Check sheet for the modelled part. Datum: model origin and axes. Units: mm. Round coordinates to 2 decimals unless told otherwise and drop trailing zeros. Loops run counter-clockwise (first coordinate to the right, second up) from the corner with the lowest first, then second, coordinate; pieces in that order, holes last. Notation, with made-up numbers: (71.5, -36) - (115.5, -36) arc R22 cw to (115.5, -2) - close; hole circle Ø6 at (-15.75, 38). An arc over 180 degrees is marked (long way). Answer in a Markdown table with one row per item. Add a question column.
(1) Thickness scan on line 1 along Y through (x, z) = (457, -11); line 2 along Y through (x, z) = (-60.5, -6.5); line 3 along X through (y, z) = (8.5, 6). Record the ranges inside material, lowest first.
(2) Gauge pin test, flat ends, axial feed: pin 1 (14.5 mm diameter, centred on x = -77, z = -15.5, fed in from +Y); pin 2 (3 mm diameter, centred on x = 212, y = 13, fed in from -Z); pin 3 (4 mm diameter, centred on y = 33, z = 10, fed in from -X). Record the tip position at first contact, or that the pin passes through.
(3) Cross-section at A-A on x = -276.5. Enter the section's corners in (y, z).
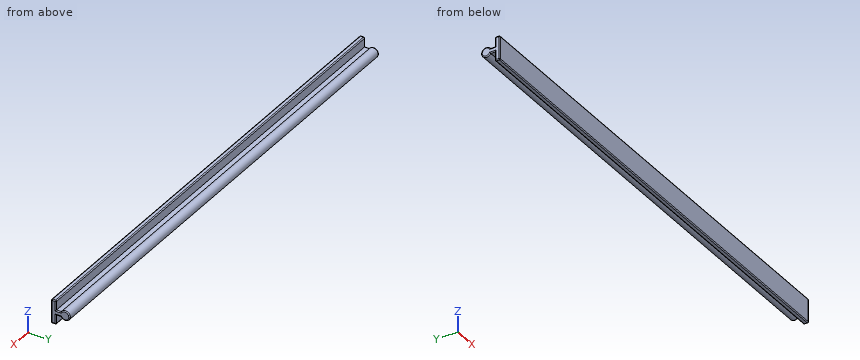
from build123d import *

# Parameters (mm, degrees)
BOSS_EXTRUDE1_DEPTH = 500
FILLET1_R           = 2


with BuildPart() as part:
    # Sketch2 → Boss-Extrude1 (new body, symmetric)
    with BuildSketch(Plane(origin=(0, 0, 0), x_dir=(0, 0, -1), z_dir=(1, 0, 0))):
        with BuildLine():
            Line((25, 0), (-25, 0))
            Line((-25, 0), (-25, 10))
            Line((-25, 10), (-5, 10))
            Line((-5, 10), (-5, 20))
            ThreePointArc((-5, 20), (0, 38.660254038), (5, 20))
            Line((5, 20), (5, 10))
            Line((5, 10), (25, 10))
            Line((25, 10), (25, 0))
        make_face()
    extrude(amount=BOSS_EXTRUDE1_DEPTH, both=True)

    # Fillet1
    fillet1_edges = [part.edges().sort_by_distance(p)[0] for p in [
        (500, 38.660254038, 0),
        (-500, 15, -5),
        (-500, 10, -15),
        (500, 15, 5),
        (0, 10, -25),
        (0, 0, -25),
        (0, 0, 25),
        (0, 10, 25),
        (500, 10, 15),
        (500, 5, 25),
        (500, 0, 0),
        (500, 5, -25),
        (500, 10, -15),
        (500, 15, -5),
        (-500, 5, -25),
        (-500, 0, 0),
        (-500, 5, 25),
        (-500, 10, 15),
        (-500, 15, 5),
        (-500, 38.660254038, 0),
    ]]
    fillet(fillet1_edges, radius=FILLET1_R)


solid = part.part
Answers:
| question | item | result |
|---|---|---|
| 1 | line 1 | y = 0 to 10 |
| 1 | line 2 | y = 0 to 10, 21.06 to 36.26 |
| 1 | line 3 | x = -499.94 to 499.94 |
| 2 | pin 1 | stops at y = 34.31 |
| 2 | pin 2 | stops at z = -5 |
| 2 | pin 3 | stops at x = -499.79 |
| 3 | outline | (0, -23) arc R2 ccw to (2, -25) - (8, -25) arc R2 ccw to (10, -23) - (10, -5) - (20, -5) arc R10 ccw (long way) to (20, 5) - (10, 5) - (10, 23) arc R2 ccw to (8, 25) - (2, 25) arc R2 ccw to (0, 23) - close |
